For this review, use the dimensioned drawing (mm, ordinates from the lowest corner) and the shaded views. Coordinates: 2 decimals unless noted, no trailing zeros. Loops run counter-clockwise (first coordinate to the right, second up) from the corner with the lowest first, then second, coordinate; pieces in that order, holes last. Notation, with made-up numbers: (26.25, 7.25) - (61.25, 7.25) arc R15 cw to (61.25, 36.25) - close; hole circle Ø2 at (-36.75, 79.5). An arc over 180 degrees is marked (long way). Use a Markdown table: item, result. Add a question column.
1) Add section A-A, the plane z = 185. Give the boundary of the cut face in (x, y), and give its area (3 significant figures).
2) To check wall thickness, follow L1, parallel to X at y = 2.55, z = 15; L2, parallel to X at y = 3.7, z = 15.5; L3, parallel to Z at x = 63, y = 2.5. State the ranges of each line that lie inside material, in increasing order. Write a range as [from, to].
3) Add section C-C, the plane z = 88. Give the boundary of the cut face in (x, y).
4) Add section D-D, the plane y = 2.5. Give the boundary of the cut face in (x, z).
5) Clearance check with a flat-ended pin moving along its axis: pin 1 (4.5 mm diameter, centred on x = 15, z = 185, fed in from +Y). State where the tip first meets the part, or that it passes through.
6) Add section B-B, the plane x = 185. Give the boundary of the cut face in (y, z).
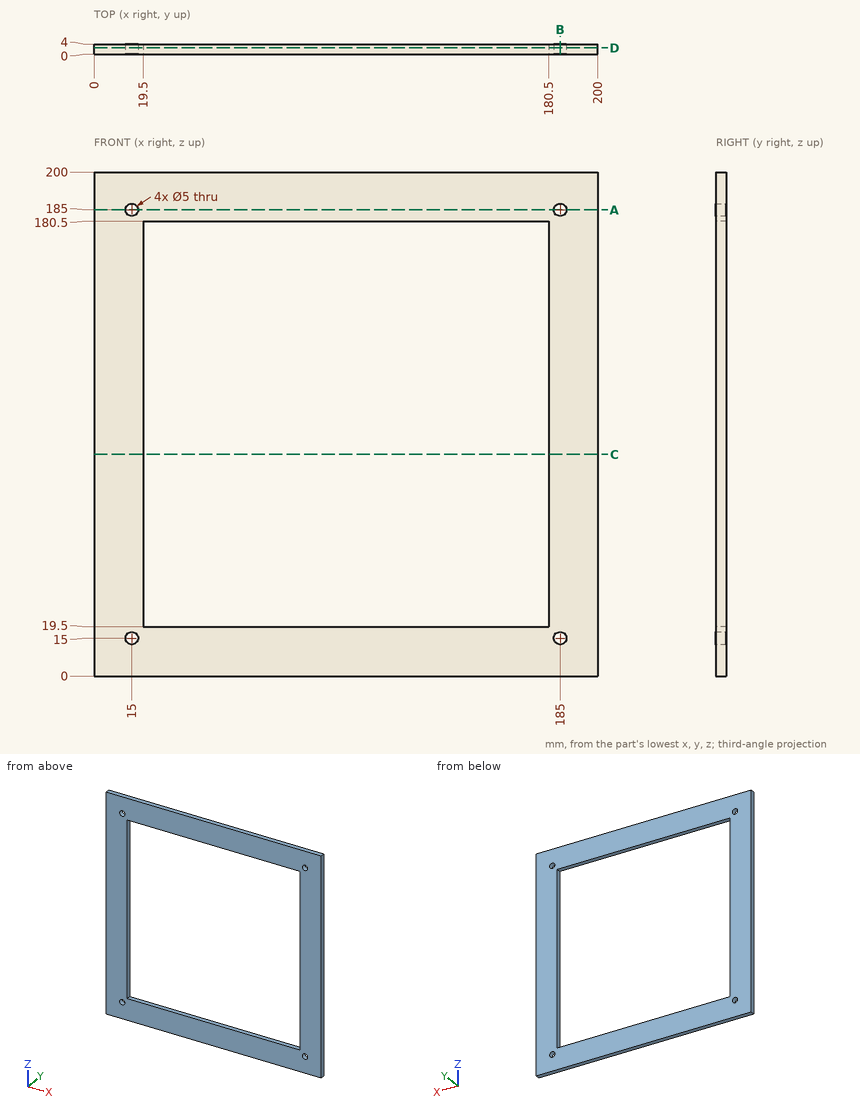
From the geometry:
| question | item | result |
|---|---|---|
| 1 | outline | (0, 0) - (12.5, 0) - (12.5, 4) - (0, 4) - close; (17.5, 0) - (182.5, 0) - (182.5, 4) - (17.5, 4) - close; (187.5, 0) - (200, 0) - (200, 4) - (187.5, 4) - close |
| 1 | area | 760 mm^2 |
| 2 | L1 | x = [0, 12.5], [17.5, 182.5], [187.5, 200] |
| 2 | L2 | x = [0, 12.55], [17.45, 182.55], [187.45, 200] |
| 2 | L3 | z = [0, 19.5], [180.5, 200] |
| 3 | outline | (0, 0) - (19.5, 0) - (19.5, 4) - (0, 4) - close; (180.5, 0) - (200, 0) - (200, 4) - (180.5, 4) - close |
| 4 | outline | (0, 0) - (200, 0) - (200, 200) - (0, 200) - close; hole circle Ø5 at (15, 15); hole circle Ø5 at (15, 185); hole (19.5, 19.5) - (180.5, 19.5) - (180.5, 180.5) - (19.5, 180.5) - close; hole circle Ø5 at (185, 15); hole circle Ø5 at (185, 185) |
| 5 | pin 1 | passes through |
| 6 | outline | (0, 0) - (4, 0) - (4, 12.5) - (0, 12.5) - close; (0, 17.5) - (4, 17.5) - (4, 182.5) - (0, 182.5) - close; (0, 187.5) - (4, 187.5) - (4, 200) - (0, 200) - close |
